Input: dimensioned drawing with shaded views. Units: mm. Origin: part minimum x, y, z. Coordinates: 2 decimals unless noted, no trailing zeros. Order: outer loops, then holes, each group sorted by start corner. A loop starts at its lowest first (then second) coordinate and runs counter-clockwise, first axis right, second up. Notation, with made-up numbers: (12, 32.5) - (55, 32.5) arc R11 ccw to (55, 37.5) - close; hole circle Ø3 at (73, 43). An arc over 180 degrees is marked (long way). Use one line per item in the form item = value. Start each with the question number.
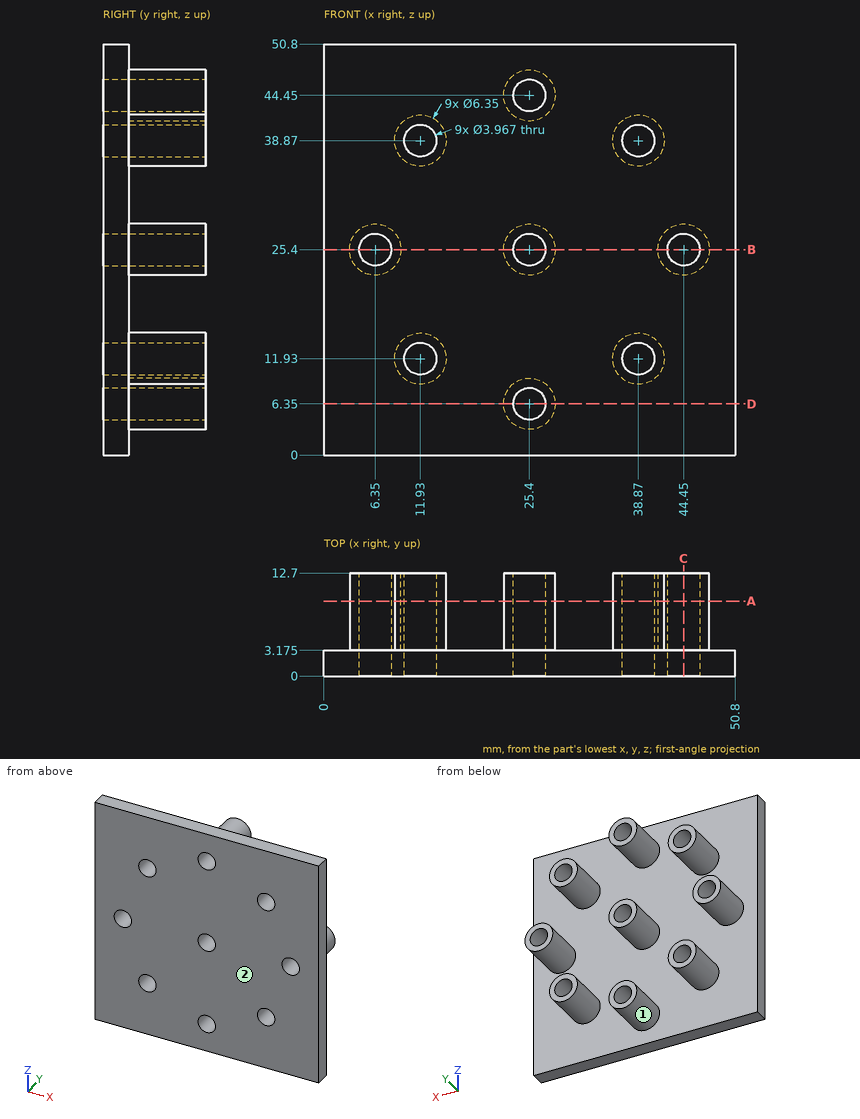
(1) Cut plane C-C on x = 44.45. Return the cut outline in (y, z) (1 decimal).
(2) Cut plane D-D on z = 6.35. Return the cut outline in (x, y) (1 decimal).
(3) Contact query for flat-ended pins moving along their axis: pin 1 Ø6 at (y, z) = (8.5, 37.5) entering from +X (1 decimal); pin 2 Ø3 at (x, z) = (11.93, 38.87) entering from +Y (3 decimals); pin 3 Ø1.5 at (x, y) = (39.5, 10) entering from -Z (1 decimal). Output: stop coordinate, or through.
(4) Cut plane A-A on y = 9.25. Count the separate pieces of the cut face and the enclosed holes in it.
(5) Material intervals for L1, parallel to Z at x = 25.4, y = 7.75 (1 decimal); L2, parallel to Z at x = 6.5, y = 11.25; L3, parallel to X at y = 0.5, z = 24.5, sorted ascending. Write a range as from..to.
(6) Cut plane B-B on z = 25.4. Return the cut outline in (x, y) (1 decimal).
(7) Draft query along Z for the marked faces 1 and 2. Return one class per face: released by +Z, released by -Z, zero draft, split by the parting line, or undercut.
Check sheet entries:
q1.outline = (0, 0) - (3.2, 0) - (3.2, 22.2) - (12.7, 22.2) - (12.7, 23.4) - (0, 23.4) - close; (0, 27.4) - (12.7, 27.4) - (12.7, 28.6) - (3.2, 28.6) - (3.2, 50.8) - (0, 50.8) - close
q2.outline = (0, 0) - (23.4, 0) - (23.4, 12.7) - (22.2, 12.7) - (22.2, 3.2) - (0, 3.2) - close; (27.4, 0) - (50.8, 0) - (50.8, 3.2) - (28.6, 3.2) - (28.6, 12.7) - (27.4, 12.7) - close
q3.pin_1 = 42
q3.pin_2 = through
q3.pin_3 = 8.8
q4.separate_pieces = 9
q4.enclosed_holes = 9
q5.L1 = 3.2..4.4, 8.3..9.5, 22.2..23.4, 27.4..28.6, 41.3..42.5, 46.4..47.6
q5.L2 = 22.23..23.42, 27.38..28.57
q5.L3 = 0..4.58, 8.12..23.63, 27.17..42.68, 46.22..50.8
q6.outline = (0, 0) - (4.4, 0) - (4.4, 12.7) - (3.2, 12.7) - (3.2, 3.2) - (0, 3.2) - close; (8.3, 0) - (23.4, 0) - (23.4, 12.7) - (22.2, 12.7) - (22.2, 3.2) - (9.5, 3.2) - (9.5, 12.7) - (8.3, 12.7) - close; (27.4, 0) - (42.5, 0) - (42.5, 12.7) - (41.3, 12.7) - (41.3, 3.2) - (28.6, 3.2) - (28.6, 12.7) - (27.4, 12.7) - close; (46.4, 0) - (50.8, 0) - (50.8, 3.2) - (47.6, 3.2) - (47.6, 12.7) - (46.4, 12.7) - close
q7.face_1 = undercut
q7.face_2 = zero draft
